Part model, mm, in its own coordinate system. A direction names the side the tool comes from. Round coordinates to 2 decimals unless told otherwise and drop trailing zeros. Write each loop counter-clockwise with the first axis right and the second up, starting at its lowest first coordinate (ties: lowest second). Pieces come first, ordered by that corner, then holes. Notation, with made-up numbers: M 79.5,-36.5 L 90.5,-36.5 A16 ccw 90.5,-5.5 Z; hole C 42.5,4.5 d11. An arc over 180 degrees is marked long. Use one line per item in the form item = value. Start each with the question number.
Item 1: Cut at B-B, the plane x = -73.5. Give the cut face in (y, z), then the cut area to 3 significant figures.
Item 2: Which spindle directions (+Z, -Z, +X, -X, +Y, -Y) get a long thin tool onto all of the face, cutting with end or side? Do faces 1 (the face through (-4, -247, -13)), 2 (the face through (-4, 3, 0)). Say none if no direction does.
Item 3: Mould opens along Y. For faces 3 (the face through (300, 1, 1)), 4 (the face through (4, 247, -13)), 5 (the face through (-4, -245, -13)), 6 (the face through (4, 245, -13)) say: +Y half, -Y half, draft (parallel to the pull), parting line (faces both ways), or undercut.
Item 4: Cut at A-A, the plane z = -13.5. Give the cut face in (x, y).
Item 5: Cut at C-C, the plane y = -206.5. Give the cut face in (x, z), then the cut area to 3 significant figures.
Item 6: Probe L1, parallel to Y at x = -219, z = -6.5; L2, parallel to Z at x = -42, y = -5.5. List the from-to ranges inside material, lowest first.
Autodesk Inventor part; units mm, degrees
ref_plane "YZ Plane" through (0, 0, 0) normal (1, 0, 0) x (0, 1, 0)
ref_plane "XZ Plane" through (0, 0, 0) normal (0, 1, 0) x (-1, 0, 0)
ref_plane "XY Plane" through (0, 0, 0) normal (0, 0, 1) x (1, 0, 0)
sketch "Sketch1" plane through (0, 0, 0) normal (0, 0, 1) x (1, 0, 0)
  line L0 (-300, -245) -> (300, -245)
  line L1 (300, -245) -> (300, 245)
  line L2 (300, 245) -> (-300, 245)
  line L3 (-300, 245) -> (-300, -245)
  line L4 (-300, -245) -> (300, 245) construction
  line L5 (300, -245) -> (-300, 245) construction
  point P0 (0, 0)
  dimension "d0" = 600
  dimension "d1" = 490
extrude "Plate1" add sketch "Sketch1" along normal blind 2
sketch "Sketch2" plane through (0, 0, 0) normal (0, 0, -1) x (-1, 0, 0)
  line L0 (-280, 225) -> (-80, 225) construction
  line L1 (-80, 225) -> (-80, 205) construction
  line L2 (-80, 205) -> (-280, 205) construction
  line L3 (-280, 205) -> (-280, 225) construction
  line L4 (-300, 245) -> (300, 245)
  line L5 (-300, -245) -> (-300, 245)
  point P0 (0, 0)
  point P1 (-48, 100)
  point P2 (300, 245)
  point P3 (-50, 98)
  dimension "d6" = 200
  dimension "d9" = 20
  dimension "d10" = 20
  dimension "d11" = 20
mark "Mark1"
sketch "Sketch3" plane through (-300, 247, 2) normal (0, -1, 0) x (1, 0, 0)
  line L0 (600, 0) -> (0, 0)
  line L1 (0, 0) -> (0, 25)
  line L2 (0, 25) -> (600, 25)
  line L3 (600, 25) -> (600, 0)
edge flange "Flange1" height 25 angle 90 thickness 2 bend radius 2.75 thickness toward (0, -1, 0) relief round relief width 2 relief depth 1 corner gap 2.75 corner form 0 edges at (0, 245, 2) (0, -245, 2) wall of the first edge with corners at (300, 247, 2) (-300, 247, 2) (-300, 247, -23) (300, 247, -23)
bend "Bend1"
corner "Corner1"
equation "\"d2\" = Thickness"
equation "\"d12\" = BendReliefWidth"
equation "\"d13\" = BendReliefDepth"
equation "\"d14\" = MinimumRemnant"
equation "\"d15\" = TransitionRadius"
equation "\"d18\" = BendRadius"
equation "\"d19\" = CornerReliefSize"
equation "\"d20\" = GapSize"
equation "\"d21\" = JacobiRadiusSize"
equation "\"BendReliefWidth\" = Thickness"
equation "\"BendReliefDepth\" = 0.5 * Thickness"
equation "\"CornerReliefSize\" = 4 * Thickness"
equation "\"MinimumRemnant\" = 2 * Thickness"
equation "\"TransitionRadius\" = BendRadius"
equation "\"JacobiRadiusSize\" = BendRadius"
equation "\"GapSize\" = Thickness"
properties part number "TRM 025 left board damper" material "AISI 304"
Model answer:
q1.outline = M -247,-23 L -245,-23 L -245,-2.75 A2.75 cw -242.25,0 L 242.25,0 A2.75 cw 245,-2.75 L 245,-23 L 247,-23 L 247,-2.75 A4.75 ccw 242.25,2 L -242.25,2 A4.75 ccw -247,-2.75 Z
q1.area = 1,070 mm²
q2.face_1 = +Z, -Z, +X, -X, -Y
q2.face_2 = -Z, +X, -X
q3.face_3 = draft
q3.face_4 = +Y half
q3.face_5 = undercut
q3.face_6 = undercut
q4.outline = M -300,-247 L 300,-247 L 300,-245 L -300,-245 Z; M -300,245 L 300,245 L 300,247 L -300,247 Z
q5.outline = M -300,0 L 300,0 L 300,2 L -300,2 Z
q5.area = 1,200 mm²
q6.L1 = -247 to -245, 245 to 247
q6.L2 = 0 to 2
